from build123d import *

# Parameters (mm, degrees)
BOSS_EXTRUDE1_DEPTH    = 7.5
BOSS_EXTRUDE2_START    = -7.5
SKETCH1_3_W            = 44.5
SKETCH1_3_H            = 36.5
BOSS_EXTRUDE2_DEPTH    = 5
BOSS_EXTRUDE3_DEPTH    = 2.5
BOSS_EXTRUDE4_DEPTH    = 5
CUT_EXTRUDE1_START     = -5
CUT_EXTRUDE1_DEPTH     = 3
M2_5_CLEARANCE_HOLE1_D = 2.9
MIRROR1_START          = -16.25
MIRROR1_DEPTH          = 3
MIRROR1_START_2        = -18.25
MIRROR1_2_OUTLINE_R    = 1.45
MIRROR1_2_DEPTH        = 2
MIRROR1_3_DEPTH        = 3
MIRROR1_START_3        = 22.25
MIRROR1_4_DEPTH        = 2.5
FILLET1_R              = 1
FILLET2_R              = 1
FILLET6_R              = 1
FILLET7_R              = 1
FILLET8_R              = 1


with BuildPart() as part:
    # Sketch1 → Boss-Extrude1 (new, symmetric)
    with BuildSketch(Plane(origin=(0, 0, 0), x_dir=(1, 0, 0), z_dir=(0, 1, 0))):
        Polygon((22.25, -18.25), (-22.25, -18.25), (-22.25, 18.25), (-24.75, 18.25), (-24.75, -20.75), (24.75, -20.75), (24.75, 18.25), (22.25, 18.25), align=None)
    extrude(amount=BOSS_EXTRUDE1_DEPTH, both=True)

    # Sketch1<3> → Boss-Extrude2 (add)
    with BuildSketch(Plane(origin=(0, 0, 0), x_dir=(1, 0, 0), z_dir=(0, 1, 0)).offset(BOSS_EXTRUDE2_START)):
        Rectangle(SKETCH1_3_W, SKETCH1_3_H)
    extrude(amount=BOSS_EXTRUDE2_DEPTH)

    # Sketch5 → Boss-Extrude3 (add)
    with BuildSketch(Plane(origin=(-24.75, 32.25, 0), x_dir=(0, 1, 0), z_dir=(-1, 0, 0))):
        Polygon((-47.15, 18.25), (-39.75, 18.25), (-39.75, -20.75), (-47.15, 13.25), align=None)
    extrude(amount=-BOSS_EXTRUDE3_DEPTH)

    # Sketch6 → Boss-Extrude4 (add)
    with BuildSketch(Plane(origin=(0, 0, -18.25), x_dir=(-1, 0, 0), z_dir=(0, 0, -1))):
        Polygon((-12.75, -10.3), (-14.266838493, -10.3), (-15.883419246, -13.1), (-19.116580754, -13.1), (-20.733161507, -10.3), (-19.116580754, -7.5), (-22.25, -7.5), (-22.25, -14.9), (-12.75, -14.9), align=None)
        Polygon((22.25, -7.5), (12.75, -7.5), (12.75, -10.3), (12.75, -14.9), (22.25, -14.9), align=None)
    extrude(amount=-BOSS_EXTRUDE4_DEPTH)

    # Sketch6<3> → Cut-Extrude1 (cut)
    with BuildSketch(Plane(origin=(0, 0, -18.25), x_dir=(-1, 0, 0), z_dir=(0, 0, -1)).offset(CUT_EXTRUDE1_START)):
        Polygon((19.0011107, -7.7), (15.9988893, -7.7), (14.4977786, -10.3), (15.9988893, -12.9), (19.0011107, -12.9), (20.5022214, -10.3), align=None)
    extrude(amount=CUT_EXTRUDE1_DEPTH, mode=Mode.SUBTRACT)

    # M2.5 Clearance Hole1 (through all)
    with Locations(Plane.XY.offset(-16.25)):
        with Locations((-17.5, -10.3), (17.5, -10.3)):
            Hole(M2_5_CLEARANCE_HOLE1_D / 2)

    # Mirror1: read off the stored shape, not the designer's step
    # Mirror1 outline → Mirror1 (cut)
    with BuildSketch(Plane.XY.offset(MIRROR1_START)):
        Polygon((-14.266838493, -10.3), (-15.883419246, -7.5), (-19.116580754, -7.5), (-20.733161507, -10.3), (-19.116580754, -13.1), (-15.883419246, -13.1), align=None)
        Polygon((-15.9988893, -12.9), (-19.0011107, -12.9), (-20.5022214, -10.3), (-19.0011107, -7.7), (-15.9988893, -7.7), (-14.4977786, -10.3), align=None, mode=Mode.SUBTRACT)
    extrude(amount=MIRROR1_DEPTH, mode=Mode.SUBTRACT)

    # Mirror1 2 outline → Mirror1 2 (add)
    with BuildSketch(Plane.XY.offset(MIRROR1_START_2)):
        Polygon((20.733161507, -10.3), (19.116580754, -7.5), (12.75, -7.5), (12.75, -10.3), (14.266838493, -10.3), (15.883419246, -13.1), (19.116580754, -13.1), align=None)
        with Locations((17.5, -10.3)):
            Circle(MIRROR1_2_OUTLINE_R, mode=Mode.SUBTRACT)
    extrude(amount=MIRROR1_2_DEPTH)

    # Mirror1 3 outline → Mirror1 3 (add)
    with BuildSketch(Plane.XY.offset(MIRROR1_START)):
        Polygon((20.733161507, -10.3), (19.116580754, -7.5), (12.75, -7.5), (12.75, -10.3), (14.266838493, -10.3), (15.883419246, -13.1), (19.116580754, -13.1), align=None)
        Polygon((15.9988893, -7.7), (19.0011107, -7.7), (20.5022214, -10.3), (19.0011107, -12.9), (15.9988893, -12.9), (14.4977786, -10.3), align=None, mode=Mode.SUBTRACT)
    extrude(amount=MIRROR1_3_DEPTH)

    # Mirror1 4 outline → Mirror1 4 (add)
    with BuildSketch(Plane.YZ.offset(MIRROR1_START_3)):
        Polygon((-14.9, -13.25), (-14.9, -18.25), (-7.5, -18.25), (-7.5, 20.75), align=None)
    extrude(amount=MIRROR1_4_DEPTH)

    # Fillet1
    fillet1_edges = [part.edges().sort_by_distance(p)[0] for p in [
        (22.25, 7.5, 0),
        (-22.25, 2.5, -18.25),
        (-22.25, 2.5, 18.25),
        (22.25, 2.5, 18.25),
        (22.25, 2.5, -18.25),
        (0, 7.5, 18.25),
        (-22.25, 7.5, 0),
        (-22.25, -2.5, 0),
        (0, -2.5, -18.25),
        (0, -2.5, 18.25),
        (22.25, -2.5, 0),
    ]]
    fillet(fillet1_edges, radius=FILLET1_R)

    # Fillet2
    fillet2_edges = [part.edges().sort_by_distance(p)[0] for p in [
        (24.75, -14.9, -15.75),
        (24.75, -11.2, 3.75),
        (24.75, 0, 20.75),
        (-24.75, 0, 20.75),
        (-24.75, -3.7, -18.25),
        (24.75, -3.7, -18.25),
        (-24.75, 7.5, 1.25),
        (-24.75, -14.9, -15.75),
        (-24.75, -11.2, 3.75),
        (24.75, 7.5, 1.25),
    ]]
    fillet(fillet2_edges, radius=FILLET2_R)

    # Fillet6
    fillet6_edges = [part.edges().sort_by_distance(p)[0] for p in [
        (-12.75, -14.9, -15.75),
        (12.75, -14.9, -15.75),
        (12.75, -11.2, -13.25),
    ]]
    fillet(fillet6_edges, radius=FILLET6_R)

    # Fillet7
    # the kernel refuses this fillet: 1 mm, written as the material it takes off along each edge
    with BuildSketch(Plane(origin=(23.75, 6.5, 19.75), x_dir=(0, 0, 1), z_dir=(0, 1, 0))) as fillet7_piece_1_section:
        Polygon((0, 0), (FILLET7_R, 0), (FILLET7_R, FILLET7_R), (0, FILLET7_R), align=None)
    fillet7_piece_1 = extrude(amount=FILLET7_R, mode=Mode.PRIVATE)
    fillet7_piece_1 = fillet7_piece_1 - Plane(origin=(23.75, 6.5, 19.75), x_dir=(-0.7071067811865476, 0, -0.7071067811865475), z_dir=(0, 1, 0)) * Sphere(FILLET7_R, mode=Mode.PRIVATE)
    add(fillet7_piece_1, mode=Mode.SUBTRACT)
    with BuildSketch(Plane(origin=(-23.75, 6.5, 19.75), x_dir=(0, 0, 1), z_dir=(0, 1, 0))) as fillet7_piece_2_section:
        Polygon((0, 0), (FILLET7_R, 0), (FILLET7_R, -FILLET7_R), (0, -FILLET7_R), align=None)
    fillet7_piece_2 = extrude(amount=FILLET7_R, mode=Mode.PRIVATE)
    fillet7_piece_2 = fillet7_piece_2 - Plane(origin=(-23.75, 6.5, 19.75), x_dir=(0.7071067811865475, 0, -0.7071067811865475), z_dir=(0, 1, 0)) * Sphere(FILLET7_R, mode=Mode.PRIVATE)
    add(fillet7_piece_2, mode=Mode.SUBTRACT)
    with BuildSketch(Plane(origin=(-23.75, 7.5, 20.75), x_dir=(0, 0, -1), z_dir=(1, 0, 0))) as fillet7_piece_3:
        with BuildLine():
            CenterArc((FILLET7_R, -FILLET7_R), FILLET7_R, 90, 90)
            Line((0, -FILLET7_R), (0, 0))
            Line((0, 0), (FILLET7_R, 0))
        make_face()
    extrude(amount=47.5, mode=Mode.SUBTRACT)

    # Fillet8
    fillet8_edges = [part.edges().sort_by_distance(p)[0] for p in [
        (22.25, -11.2, 3.75),
        (-22.25, -11.2, 3.75),
    ]]
    fillet(fillet8_edges, radius=FILLET8_R)


solid = part.part
Can you work these out from the model? Positions are in its coordinate system, mm. A direction names the side the tool comes from. Coordinates: 2 decimals unless noted, no trailing zeros. Write each loop counter-clockwise with the first axis right and the second up, starting at its lowest first coordinate (ties: lowest second). Pieces come first, ordered by that corner, then holes. Notation, with made-up numbers: (-34, 1.5) - (16, 1.5) arc R18 cw to (16, 8.5) - close; hole circle Ø1 at (73.5, 54.25). An arc over 180 degrees is marked (long way). Return JSON: item names as keys, results as strings. Group by question number.
Item 1: Which directions (+Z, -Z, +X, -X, +Y, -Y) give clear straight access to the entire face, cutting with the end or side of a thin tool? Please do faces 1 (the face through (-12.75, -11, -16)), 2 (the face through (19.5, -12.8, -13.25)), 3 (the face through (19.762, -11.582, -14.771)).
Item 2: If we section it at A-A (x = -17.5): Write out the boundary of the cut face in (y, z).
Item 3: I'm going to push flat-ended pins straight in: pin 1 Ø2 at (x, y) = (-16.5, -11.5) entering from +Z; pin 2 Ø2.5 at (x, y) = (17.5, -10.3) entering from +Z; pin 3 Ø5 at (x, z) = (2, -4.5) entering from -Y; pin 4 Ø1.5 at (x, z) = (16.5, -11) entering from +Y. Where does each tip first touch, or does it pass through?
Item 4: If we section it at D-D (x = 17.5): Write out the boundary of the cut face in (y, z).
Item 5: We'd pull the mould along X, two halves only. Please class faces 4 (the face through (19, -14.9, -16)), 5 (the face through (-15.064, -8.92, -14.771)), 6 (the face through (-24.46, -10.96, 3.45)): pulls with the +X half, pulls with the -X half, needs draft (parallel to the pull), parting line crosses it, or undercut.
Item 6: If we section it at B-B (x = 5): Write out the boundary of the cut face in (y, z).
Item 7: Please list where these lines run through material, in increasing order: probe 1 along Y at (x, z) = (17, -16); probe 2 along X at (y, z) = (-9.5, -9.5); probe 3 along Y at (x, z) = (17.5, -16.85).
Item 8: If we section it at C-C (y = 3.5): Write out the boundary of the cut face in (x, z).
Return value:
{
 "1": {"face 1": "+Z, -Z, -Y", "face 2": "+Z, -Y", "face 3": "+Z"},
 "2": {"outline": "(-14.9, -18.25) - (-11.75, -18.25) - (-11.75, -16.25) - (-13.1, -16.25) - (-13.1, -13.25) - (-14.9, -13.25) - close; (-8.85, -18.25) - (-3.5, -18.25) arc R1 ccw to (-2.5, -17.25) - (-2.5, 17.25) arc R1 cw to (-1.5, 18.25) - (6.5, 18.25) arc R1 ccw to (7.5, 19.25) - (7.5, 19.75) arc R1 ccw to (6.5, 20.75) - (-7.5, 20.75) - (-7.5, -16.25) - (-8.85, -16.25) - close"},
 "3": {"pin 1": "stops at z = -16.25", "pin 2": "passes through", "pin 3": "stops at y = -7.5", "pin 4": "stops at y = -2.5"},
 "4": {"outline": "(-14.9, -18.25) - (-11.75, -18.25) - (-11.75, -16.25) - (-12.9, -16.25) - (-12.9, -13.25) - (-14.9, -13.25) - close; (-8.85, -18.25) - (-3.5, -18.25) arc R1 ccw to (-2.5, -17.25) - (-2.5, 17.25) arc R1 cw to (-1.5, 18.25) - (6.5, 18.25) arc R1 ccw to (7.5, 19.25) - (7.5, 19.75) arc R1 ccw to (6.5, 20.75) - (-7.5, 20.75) - (-7.5, -13.25) - (-7.7, -13.25) - (-7.7, -16.25) - (-8.85, -16.25) - close"},
 "5": {"face 4": "needs draft", "face 5": "undercut", "face 6": "pulls with the -X half"},
 "6": {"outline": "(-7.5, -18.25) - (-3.5, -18.25) arc R1 ccw to (-2.5, -17.25) - (-2.5, 17.25) arc R1 cw to (-1.5, 18.25) - (6.5, 18.25) arc R1 ccw to (7.5, 19.25) - (7.5, 19.75) arc R1 ccw to (6.5, 20.75) - (-7.5, 20.75) - close"},
 "7": {"probe 1": "y = -14.9 to -12.9, -7.7 to -2.5", "probe 2": "x = -24.75 to -22.25, 22.25 to 24.75", "probe 3": "y = -14.9 to -11.75, -8.85 to -2.5"},
 "8": {"outline": "(-24.75, -17.25) arc R1 ccw to (-23.75, -18.25) - (-23.25, -18.25) arc R1 ccw to (-22.25, -17.25) - (-22.25, 17.25) arc R1 cw to (-21.25, 18.25) - (21.25, 18.25) arc R1 cw to (22.25, 17.25) - (22.25, -17.25) arc R1 ccw to (23.25, -18.25) - (23.75, -18.25) arc R1 ccw to (24.75, -17.25) - (24.75, 19.75) arc R1 ccw to (23.75, 20.75) - (-23.75, 20.75) arc R1 ccw to (-24.75, 19.75) - close"}
}
